For this review, take the finished solid that the model builds, in its own axes (mm). Face numbers are marked on the shaded views. Round coordinates to 2 decimals unless told otherwise and drop trailing zeros. Loops run counter-clockwise (first coordinate to the right, second up) from the corner with the lowest first, then second, coordinate; pieces in that order, holes last. Notation, with made-up numbers: (-38, 67) -> (10, 67) arc R22 ccw to (10, 92) -> close; hole circle Ø9 at (-11, 29). An arc over 180 degrees is marked (long way). One line per question, with ' | ' between items. Start each with the question number.
1. Consider section C-C (y = 6.25). Count the separate pieces of the cut face and the enclosed holes in it, and give its area (3 significant figures).
2. For pin 1 Ø8.5 at (x, z) = (147, -172) entering from -Y; pin 2 Ø4 at (x, z) = (160, -6.1) entering from -Y; pin 3 Ø2.5 at (y, z) = (4, -10) entering from -X, all flat-tipped, find the tip position at first contact; note any pin that passes through.
3. Wall thickness on line 1 along X through (y, z) = (6, -6.1); line 2 along Z through (x, y) = (64.9, 3.2); line 3 along Z through (x, y) = (95, 5.5): over which ranges is each line inside the solid? List them lowest first.
4. Consider section A-A (z = -49.5). Write out the cut boundary in (x, y), and give its area (3 significant figures).
5. Draft analysis for pull direction X (two halves, no side actions). For the marked faces 1 and 2, state which applies: pulls with the +X half, pulls with the -X half, needs draft (parallel to the pull), parting line crosses it, or undercut.
6. Consider section B-B (x = 83.5). Write out the cut boundary in (y, z).
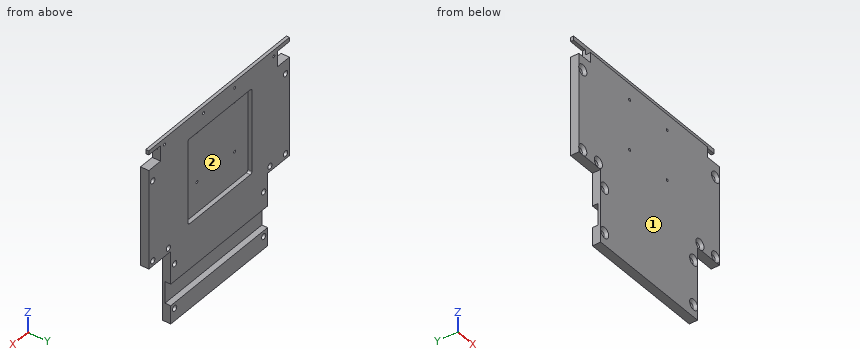
Autodesk Inventor part; units mm, degrees
ref_plane "YZ Plane" through (0, 0, 0) normal (1, 0, 0) x (0, 1, 0)
ref_plane "XZ Plane" through (0, 0, 0) normal (0, 1, 0) x (-1, 0, 0)
ref_plane "XY Plane" through (0, 0, 0) normal (0, 0, 1) x (1, 0, 0)
sketch "Sketch1" plane through (0, 0, 0) normal (0, 1, 0) x (-1, 0, 0)
  line L0 (0, 0) -> (-180, 0)
  line L1 (0, 0) -> (0, -4)
  line L2 (0, -4) -> (-15, -4)
  line L3 (-15, -4) -> (-15, -19)
  line L4 (-15, -19) -> (0, -19)
  line L5 (-180, -4) -> (-165, -4)
  line L6 (-165, -4) -> (-165, -19)
  line L7 (-165, -19) -> (-180, -19)
  line L8 (-180, -4) -> (-180, 0)
  line L9 (0, -19) -> (0, -114)
  line L10 (0, -114) -> (-28, -114)
  line L11 (-28, -114) -> (-28, -184)
  line L12 (-28, -184) -> (-152, -184)
  line L13 (-152, -184) -> (-152, -114)
  line L14 (-152, -114) -> (-180, -114)
  line L15 (-180, -114) -> (-180, -19)
  dimension "d11" = 4
  dimension "d12" = 15
  dimension "d13" = 15
  dimension "d14" = 15
  dimension "d15" = 15
  dimension "d41" = 95
  dimension "d42" = 28
  dimension "d43" = 70
  dimension "d44" = 70
  dimension "d45" = 28
extrude "Extrusion1" add sketch "Sketch1" along normal blind 8
sketch "Sketch2" plane through (0, 0, 0) normal (0, -1, 0) x (1, 0, 0)
  line L0 (0, 0) -> (180, 0)
  line L1 (180, 0) -> (180, -9.1)
  line L2 (180, -9.1) -> (0, -9.1)
  line L3 (0, -9.1) -> (0, 0)
  dimension "d7" = 180
  dimension "d8" = 9.1
extrude "Extrusion2" cut sketch "Sketch2" against normal blind 5
sketch "Sketch6" plane through (0, 5, 0) normal (0, -1, 0) x (1, 0, 0)
  line L0 (165, -9.1) -> (15, -9.1)
  line L1 (15, -9.1) -> (15, -6.1)
  line L2 (15, -19) -> (15, -4)
  line L3 (15, -6.1) -> (20, -6.1)
  line L4 (20, -6.1) -> (70, -6.1)
  line L5 (70, -6.1) -> (110, -6.1)
  line L6 (110, -6.1) -> (160, -6.1)
  point P0 (0, 0)
  dimension "d28" = 3
  dimension "d29" = 5
  dimension "d30" = 50
  dimension "d31" = 40
  dimension "d32" = 50
hole "Hole1" at (20, 5, -6.1) at (70, 5, -6.1) at (110, 5, -6.1) at (160, 5, -6.1) direction (0, 1, 0) diameter 2.4638 end through all
sketch "Sketch7" plane through (152, 0, -114) normal (1, 0, 0) x (0, 0, -1)
  line L0 (70, 0) -> (42, 0)
  line L1 (70, 0) -> (0, 0)
  line L2 (42, 0) -> (42, 15)
  circle A0 centre (42, 15) radius 12.5
  point P0 (-114, 0)
  dimension "d46" = 28
  dimension "d47" = 15
  dimension "d48" = 25
extrude "Extrusion5" cut sketch "Sketch7" against normal blind 124
sketch "Sketch8" plane through (0, 8, 0) normal (0, 1, 0) x (1, 0, 0)
  line L0 (0, 0) -> (180, 0)
  line L1 (0, 4) -> (0, 0)
  line L2 (0, 0) -> (48, 0)
  line L3 (48, 0) -> (48, 20)
  line L4 (48, 20) -> (130, 20)
  line L5 (130, 20) -> (130, 102)
  line L6 (130, 102) -> (48, 102)
  line L7 (48, 102) -> (48, 20)
  dimension "d114" = 48
  dimension "d115" = 20
  dimension "d116" = 82
  dimension "d117" = 82
extrude "Extrusion6" cut sketch "Sketch8" against normal blind 4
sketch "Sketch11" plane through (0, 0, 0) normal (0, -1, 0) x (1, 0, 0)
  line L0 (0, -114) -> (5, -114)
  line L1 (5, -114) -> (5, -109)
  line L2 (0, -109) -> (0, -114)
  line L3 (0, -109) -> (5, -109)
  line L4 (180, -114) -> (175, -114)
  line L5 (175, -114) -> (175, -109)
  line L6 (180, -109) -> (180, -114)
  line L7 (180, -109) -> (175, -109)
  line L8 (0, -19) -> (5, -19)
  line L9 (5, -19) -> (5, -32)
  line L10 (5, -32) -> (0, -32)
  line L11 (0, -32) -> (0, -19)
  line L12 (165, -19) -> (180, -19)
  line L13 (180, -19) -> (175, -19)
  line L14 (175, -19) -> (175, -32)
  line L15 (175, -32) -> (180, -32)
  line L16 (180, -32) -> (180, -19)
  line L17 (5, -109) -> (25, -109)
  line L18 (175, -109) -> (155, -109)
  line L19 (28, -184) -> (28, -114)
  line L20 (28, -184) -> (33, -184)
  line L21 (33, -184) -> (33, -172)
  line L22 (33, -172) -> (28, -172)
  line L23 (28, -172) -> (28, -184)
  line L24 (152, -184) -> (28, -184)
  line L25 (152, -184) -> (147, -184)
  line L26 (147, -184) -> (147, -172)
  line L27 (147, -172) -> (152, -172)
  line L28 (152, -172) -> (152, -184)
  line L29 (28, -145.6438) -> (28, -114)
  line L30 (28, -114) -> (33, -114)
  line L31 (33, -114) -> (33, -129)
  line L32 (33, -129) -> (28, -129)
  line L33 (28, -129) -> (28, -114)
  line L34 (180, -114) -> (152, -114)
  line L35 (152, -114) -> (147, -114)
  line L36 (147, -114) -> (147, -129)
  line L37 (147, -129) -> (152, -129)
  line L38 (152, -129) -> (152, -114)
  point P0 (0, 0)
  point P1 (145, -19)
  dimension "d88" = 5
  dimension "d89" = 5
  dimension "d92" = 5
  dimension "d105" = 5
  dimension "d106" = 13
  dimension "d107" = 20
  dimension "d108" = 20
  dimension "d131" = 5
  dimension "d132" = 12
  dimension "d133" = 5
  dimension "d134" = 12
  dimension "d136" = 5
  dimension "d137" = 15
hole "Hole4" at (5, 0, -109) at (175, 0, -109) at (175, 0, -32) at (5, 0, -32) at (155, 0, -109) at (25, 0, -109) at (33, 0, -129) at (33, 0, -172) at (147, 0, -172) at (147, 0, -129) direction (0, 1, 0) diameter 5.4 end through all countersink diameter 10.3886 countersink angle 90
sketch "Sketch12" plane through (0, 4, 0) normal (0, 1, 0) x (1, 0, 0)
  line L0 (48, 20) -> (48, 102)
  line L1 (48, 20) -> (64.9, 20)
  line L2 (130, 20) -> (48, 20)
  line L3 (64.9, 20) -> (64.9, 24.4)
  line L4 (64.9, 24.4) -> (64.9, 72.6)
  line L5 (64.9, 24.4) -> (113.1, 24.4)
  line L6 (64.9, 24.4) -> (113.1, 72.6)
  point P0 (0, 0)
  dimension "d119" = 16.9
  dimension "d120" = 4.4
  dimension "d121" = 48.2
  dimension "d122" = 48.2
hole "Hole5" at (64.9, 4, -72.6) at (64.9, 4, -24.4) at (113.1, 4, -72.6) at (113.1, 4, -24.4) direction (0, -1, 0) diameter 2.4638 end through all
fillet "Fillet2" radius 2 4 edges at (48, 6, -102) (130, 6, -102) (130, 6, -20) (48, 6, -20)
sketch "Sketch13" plane through (152, 0, -184) normal (1, 0, 0) x (0, 0, -1)
  arc A0 (-38.3562, 8) -> (-17.6438, 8) centre (-28, 15) ccw
  circle A1 centre (-28, 15) radius 19.5
  line L0 (-174.9, 0) -> (-174.9, 5)
  line L1 (-174.9, 0) -> (-195, 0)
  line L2 (-195, 0) -> (-24.2057, -4.6095)
  point P0 (-184, 0)
  dimension "d138" = 39
  dimension "d139" = 20.1
sketch "Sketch14" plane through (0, 8, 0) normal (0, 1, 0) x (1, 0, 0)
  line L0 (152, 166.3562) -> (152, 145.6438)
  line L1 (152, 156) -> (28, 156)
  line L2 (28, 145.6438) -> (28, 166.3562)
  line L3 (28, 145.6) -> (152, 145.6)
  line L4 (152, 145.6) -> (152, 166.4)
  line L5 (152, 166.4) -> (28, 166.4)
  line L6 (28, 166.4) -> (28, 145.6)
  point P0 (0, 0)
  dimension "d140" = 20.8
extrude "Extrusion7" cut sketch "Sketch14" against normal blind 5.5
properties part number "blacha"
Answer block:
1) separate pieces: 2 | enclosed holes: 15 | area: 19,200 mm2
2) pin 1: stops at y = 0.94 | pin 2: stops at y = 5 | pin 3: stops at x = 15
3) line 1: x = 15 to 18.77, 21.23 to 68.77, 71.23 to 108.77, 111.23 to 158.77, 161.23 to 165 | line 2: z = -184 to -166.4, -145.6 to -73.83, -71.37 to -25.63, -23.17 to -9.1 | line 3: z = -184 to -166.4, -145.6 to -102, -20 to 0
4) outline: (0, 0) -> (180, 0) -> (180, 8) -> (130, 8) -> (130, 4) -> (48, 4) -> (48, 8) -> (0, 8) -> close | area: 1,110 mm2
5) face 1: needs draft | face 2: undercut
6) outline: (0, -184) -> (8, -184) -> (8, -166.4) -> (2.5, -166.4) -> (2.5, -145.6) -> (8, -145.6) -> (8, -102) -> (4, -102) -> (4, -20) -> (8, -20) -> (8, 0) -> (5, 0) -> (5, -9.1) -> (0, -9.1) -> close
